from build123d import *

# Parameters (mm, degrees)
F0_W     = 20
F0_H     = 20
F1_DEPTH = 10
F2_T     = -1


# Not quite as in the source:
# - a feature names something its author has since deleted; it is built from what else it names


with BuildPart() as f1:
    # F0 (on Top) → F1 (new body)
    with BuildSketch(Plane.XY):
        Rectangle(F0_W, F0_H)
    extrude(amount=F1_DEPTH)

    # F2 (hollow: no face is removed)
    offset(amount=F2_T, mode=Mode.SUBTRACT)


solid = f1.part
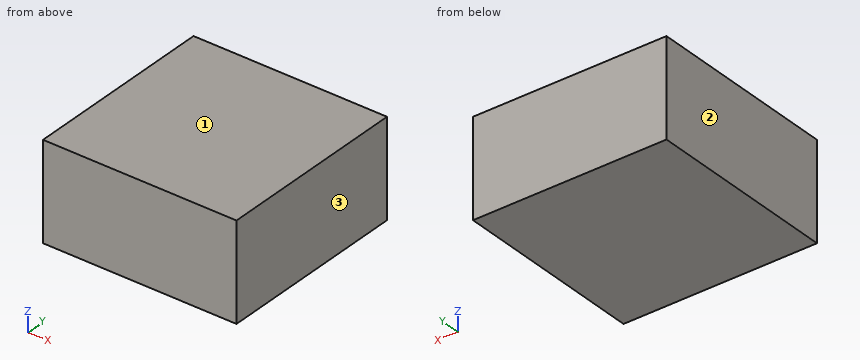
CAD build for the part. Positions are in the model's coordinates, mm. Face numbers are marked on the shaded views. Give positions to 0.01 mm unless a question says otherwise; leave off trailing zeros. Write each loop counter-clockwise with the first axis right and the second up, starting at its lowest first coordinate (ties: lowest second). Pieces come first, ordered by that corner, then holes. Notation, with made-up numbers: M -17,38.5 L 4,38.5 A27 ccw 4,64.5 Z; hole C 53,13.5 d3. An arc over 180 degrees is marked long. Put each result on its own line as item: value. Start each with the question number.
(1) Mould opens along X. For the marked faces 1, 2 and 3 say: +X half, -X half, draft (parallel to the pull), parting line (faces both ways), or undercut.
(2) Probe L1, parallel to X at y = -6.5, z = 6.75; L2, parallel to Z at x = -2, y = 7.75. List the from-to ranges inside material, lowest first.
(3) Band-saw the part on A-A, the plane z = 3. Write the cut outline in (x, y).
(4) Flat gauge pin, fed straight in: pin 1 Ø1.5 at (x, y) = (-7, 3.5) entering from -Z. Where does the tip first touch, or does it go through?
(5) Band-saw the part on B-B, the plane y = -5.5. Write the cut outline in (x, z), and give its area (3 significant figures).
Response values:
1. face 1: draft
1. face 2: -X half
1. face 3: +X half
2. L1: x = -10 to -9, 9 to 10
2. L2: z = 0 to 1, 9 to 10
3. outline: M -10,-10 L 10,-10 L 10,10 L -10,10 Z; hole M -9,-9 L 9,-9 L 9,9 L -9,9 Z
4. pin 1: stops at z = 0
5. outline: M -10,0 L 10,0 L 10,10 L -10,10 Z; hole M -9,1 L 9,1 L 9,9 L -9,9 Z
5. area: 56.0 mm2
